Can you work these out from the model? Positions are in its coordinate system, mm. Face numbers are marked on the shaded views. A direction names the side the tool comes from. Round coordinates to 2 decimals unless told otherwise and drop trailing zeros. Loops run counter-clockwise (first coordinate to the right, second up) from the corner with the lowest first, then second, coordinate; pieces in that order, holes last. Notation, with made-up numbers: M 27.5,82.25 L 81.5,82.25 A11 cw 81.5,89.25 Z; hole C 64,21 d6. An arc over 180 degrees is marked long. Use a Markdown table: item, result. Add a question column.
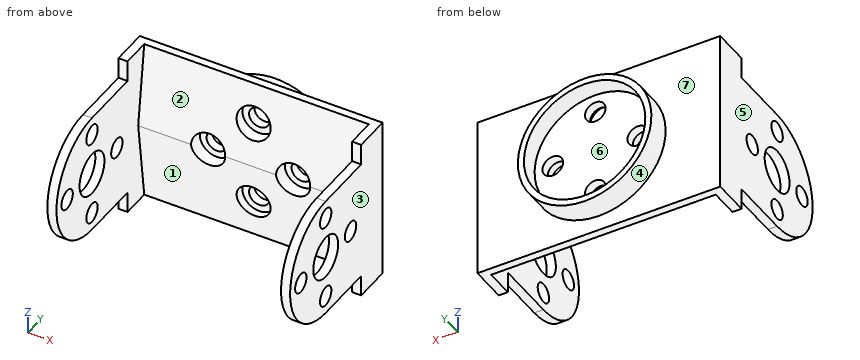
```python
from build123d import *

# Parameters (mm, degrees)
SKETCH_1_W               = 40
SKETCH_1_H               = 28
EXTRUDE_1_DEPTH          = 27
SKETCH_2_W               = 37
SKETCH_2_H               = 27
CUT_EXTRUDE_1_DEPTH      = 25
SKETCH_3_R               = 1.6
SKETCH_3_R_2             = 3.5
CUT_EXTRUDE_2_DEPTH      = 56.794264938
SKETCH_4_R               = 11
SKETCH_4_R_2             = 10
EXTRUDE_2_DEPTH          = 4
SKETCH_11_R              = 10
EXTRUDE_3_DEPTH          = 1
CUT_EXTRUDE_3_DEPTH      = 56.794264938
CUT_EXTRUDE_3_DEPTH_BACK = 56.794264938
SKETCH_6_R               = 1.7
SKETCH_7_R               = 2.8
CUT_EXTRUDE_4_DEPTH      = 2.5
CUT_EXTRUDE_6_REACH      = 58.879
CUT_EXTRUDE_5_DEPTH      = 58.905094767


with BuildPart() as part:
    # 草图1 → 凸台-拉伸1 (new body)
    with BuildSketch(Plane.XY):
        with Locations((20, 14)):
            Rectangle(SKETCH_1_W, SKETCH_1_H)
    extrude(amount=EXTRUDE_1_DEPTH)

    # 草图2 → 切除-拉伸1 (cut)
    with BuildSketch(Plane.XZ):
        with Locations((20, 13.5)):
            Rectangle(SKETCH_2_W, SKETCH_2_H)
    extrude(amount=-CUT_EXTRUDE_1_DEPTH, mode=Mode.SUBTRACT)

    # 草图3 → 切除-拉伸2 (cut, through all)
    with BuildSketch(Plane.ZY):
        with Locations((13.5, 5)):
            Circle(SKETCH_3_R)
        with Locations((13.5, 12)):
            Circle(SKETCH_3_R_2)
        with Locations((6.5, 12)):
            Circle(SKETCH_3_R)
        with Locations((20.5, 12)):
            Circle(SKETCH_3_R)
        with Locations((13.5, 19)):
            Circle(SKETCH_3_R)
    extrude(amount=-CUT_EXTRUDE_2_DEPTH, mode=Mode.SUBTRACT)

    # 草图4 → 凸台-拉伸2 (add)
    with BuildSketch(Plane(origin=(0, 28, 0), x_dir=(1, 0, 0), z_dir=(0, 1, 0))):
        with Locations(Location((20, -13.5, 0), (0, 0, 90))):
            Circle(SKETCH_4_R)
        with Locations(Location((20, -13.5, 0), (0, 0, 270))):
            Circle(SKETCH_4_R_2, mode=Mode.SUBTRACT)
    extrude(amount=EXTRUDE_2_DEPTH)

    # 草图11 → 凸台-拉伸3 (add)
    with BuildSketch(Plane(origin=(0, 28, 0), x_dir=(1, 0, 0), z_dir=(0, 1, 0))):
        with Locations(Location((20, -13.5, 0), (0, 0, 270))):
            Circle(SKETCH_11_R)
    extrude(amount=EXTRUDE_3_DEPTH)

    # 草图6 → 切除-拉伸3 (cut, two sides: drawn at the far end of the back side and taken through both)
    with BuildSketch(Plane(origin=(0, 28, 0), x_dir=(1, 0, 0), z_dir=(0, 1, 0)).offset(-CUT_EXTRUDE_3_DEPTH_BACK)):
        with Locations(Location((20, -6.5, 0), (0, 0, 270))):
            Circle(SKETCH_6_R)
        with Locations(Location((27, -13.5, 0), (0, 0, 270))):
            Circle(SKETCH_6_R)
        with Locations(Location((20, -20.5, 0), (0, 0, 270))):
            Circle(SKETCH_6_R)
        with Locations(Location((13, -13.5, 0), (0, 0, 270))):
            Circle(SKETCH_6_R)
    extrude(amount=CUT_EXTRUDE_3_DEPTH + CUT_EXTRUDE_3_DEPTH_BACK, mode=Mode.SUBTRACT)

    # 草图7 → 切除-拉伸4 (cut)
    with BuildSketch(Plane.XZ.offset(-25)):
        with Locations(Location((20, 20.5, 0), (0, 0, 270))):
            Circle(SKETCH_7_R)
        with Locations(Location((27, 13.5, 0), (0, 0, 270))):
            Circle(SKETCH_7_R)
        with Locations(Location((20, 6.5, 0), (0, 0, 270))):
            Circle(SKETCH_7_R)
        with Locations(Location((13, 13.5, 0), (0, 0, 270))):
            Circle(SKETCH_7_R)
    extrude(amount=-CUT_EXTRUDE_4_DEPTH, mode=Mode.SUBTRACT)

    # 切除-拉伸6: up to this face of the body (flat: up to its plane)
    cut_extrude_6_end = Plane(part.part.faces().sort_by_distance((38.5, 12.5, 0.36796739))[0])
    # 草图10 → 切除-拉伸6 (cut, up to the picked face)
    with BuildSketch(Plane(origin=(1.5, 0, 0), x_dir=(0, 0, -1), z_dir=(1, 0, 0)), mode=Mode.PRIVATE) as cut_extrude_6_sk1:
        Polygon((-13.5, 25), (0, 25), (0, 26.7), align=None)
    cut_extrude_6_tool1 = split(extrude(cut_extrude_6_sk1.sketch, amount=CUT_EXTRUDE_6_REACH, mode=Mode.PRIVATE), bisect_by=cut_extrude_6_end, keep=Keep.BOTH, mode=Mode.PRIVATE)
    # 草图10 → 切除-拉伸6 (cut, up to the picked face)
    with BuildSketch(Plane(origin=(1.5, 0, 0), x_dir=(0, 0, -1), z_dir=(1, 0, 0)), mode=Mode.PRIVATE) as cut_extrude_6_sk2:
        Polygon((-27, 25), (-13.5, 25), (-27, 26.7), align=None)
    cut_extrude_6_tool2 = split(extrude(cut_extrude_6_sk2.sketch, amount=CUT_EXTRUDE_6_REACH, mode=Mode.PRIVATE), bisect_by=cut_extrude_6_end, keep=Keep.BOTH, mode=Mode.PRIVATE)
    add(cut_extrude_6_tool1.solids().sort_by(Axis((1.5, 25.566667, 4.5), (1, 0, 0)))[0], mode=Mode.SUBTRACT)
    add(cut_extrude_6_tool2.solids().sort_by(Axis((1.5, 25.566667, 22.5), (1, 0, 0)))[0], mode=Mode.SUBTRACT)

    # 草图9 → 切除-拉伸5 (cut, through all)
    with BuildSketch(Plane.ZY):
        with BuildLine():
            Line((3.5, 22), (0, 22))
            Line((0, 22), (0, 0))
            Line((0, 0), (27, 0))
            Line((27, 0), (27, 22))
            Line((27, 22), (23.5, 22))
            Line((23.5, 22), (23.5, 12))
            ThreePointArc((23.5, 12), (13.5, 2), (3.5, 12))
            Line((3.5, 12), (3.5, 22))
        make_face()
    extrude(amount=-CUT_EXTRUDE_5_DEPTH, mode=Mode.SUBTRACT)


solid = part.part
```
(1) Thinking about a two-plate mould opening in X: for the marked faces 5, 6 and 7, which applies, released by +X, released by -X, zero draft, split by the parting line, or undercut?
(2) Suppose I cut it at A-A on y = 19. List the corners of the cut face in (x, z) for me.
(3) On a 3-axis mill with a long thin cutter (end or side, diameter ignored), from which of +Z, -Z, +X, -X, +Y, -Y can I reach the whole of each face in a straight line? I mean the marked faces 1, 2, 3 and 4. Say none if no direction works.
(4) If I drill on probe 1 along X at (y, z) = (25.55, 13.5); probe 2 along Z at (x, y) = (20, 26.85); probe 3 along X at (y, z) = (31, 13.5), over which ranges is the centre line in solid material (lowest first)? Write a range as [from, to].
(5) Suppose I cut it at C-C on y = 24.5. List the corners of the cut face in (x, z) for me, and give its area (3 significant figures).
(6) I'm going to push flat-ended pins straight in: pin 1 (4 mm diameter, centred on x = 27, z = 13.5, fed in from -Y); pin 2 (1.5 mm diameter, centred on x = 12.5, z = 9, fed in from +Y); pin 3 (3 mm diameter, centred on x = 17, z = 23, fed in from -Y). Where does each tip first touch, or does it pass through?
(7) Suppose I cut it at B-B on x = 19. Count the separate pieces of the cut face and the enclosed holes in it, and give its area (3 significant figures).
Results below:
| question | item | result |
|---|---|---|
| 1 | face 5 | released by -X |
| 1 | face 6 | undercut |
| 1 | face 7 | zero draft |
| 2 | outline | M 0,3.5 L 1.5,3.5 L 1.5,11.9 L 0,11.9 Z; M 0,15.1 L 1.5,15.1 L 1.5,23.5 L 0,23.5 Z; M 38.5,3.5 L 40,3.5 L 40,11.9 L 38.5,11.9 Z; M 38.5,15.1 L 40,15.1 L 40,23.5 L 38.5,23.5 Z |
| 3 | face 1 | -Z, -Y |
| 3 | face 2 | +Z, -Y |
| 3 | face 3 | +Z, -Z, +X, +Y, -Y |
| 3 | face 4 | +Y |
| 4 | probe 1 | x = [0, 10.2], [15.8, 24.2], [29.8, 40] |
| 4 | probe 2 | z = [0, 3.7], [9.3, 17.7], [23.3, 27] |
| 4 | probe 3 | x = [9, 10], [30, 31] |
| 5 | outline | M 0,0 L 1.5,0 L 1.5,27 L 0,27 Z; M 38.5,0 L 40,0 L 40,27 L 38.5,27 Z |
| 5 | area | 81.0 mm² |
| 6 | pin 1 | stops at y = 27.5 |
| 6 | pin 2 | stops at y = 29 |
| 6 | pin 3 | stops at y = 26.01 |
| 7 | separate pieces | 3 |
| 7 | enclosed holes | 0 |
| 7 | area | 60.8 mm² |
